Source: CAD feature listing. Evaluate the final solid. Frame: model axes, mm. Give positions to 0.01 mm unless a question says otherwise; leave off trailing zeros. Loops run counter-clockwise (first coordinate to the right, second up) from the corner with the lowest first, then second, coordinate; pieces in that order, holes last. Notation, with made-up numbers: (61, 44.25) -> (69, 44.25) arc R7 ccw to (69, 55.25) -> close; hole circle Ø2 at (-1.75, 14). An arc over 180 degrees is marked (long way). Return JSON: item names as keys, results as strings. Group by question number.
(1) Cut plane D-D on x = 76.2. Return loops of the section in (y, z).
(2) Cut plane C-C on z = -76.2. Return loops of the section in (x, y).
(3) Cut plane B-B on y = 1. Give the number of separate pieces and of enclosed holes in the cut face, then the cut area to 3 significant figures.
(4) Pin query (flat end, axial travel): pin 1 (3 mm diameter, centred on x = 56.5, y = 4.5, fed in from -Z); pin 2 (3 mm diameter, centred on y = 3, z = 1.5, fed in from -X); pin 3 (3 mm diameter, centred on y = 2.5, z = 12, fed in from +X). Return the tip coordinate at first contact, or that it passes through.
(5) Cut plane A-A on x = 0. Return loops of the section in (y, z).
(6) Ray query, line 1 (X direction, y = 3, z = 76.2); line 2 (Z direction, x = 1, y = 3.25); line 3 (Z direction, x = -78, y = 1). Return the intervals inside material, ascending. Write a range as from..to.
```python
from build123d import *

# Parameters (mm, degrees)
BOSS_EXTRUDE1_DEPTH         = 6.35
SKETCH2_R                   = 50.8
CUT_EXTRUDE1_DEPTH          = 6.35
FILLET1_R                   = 50.8
F_1_2_20_TAPPED_HOLE1_D     = 11.50874
F_1_2_20_TAPPED_HOLE1_DEPTH = 29.21
F_1_2_20_TAPPED_HOLE1_TIP   = 3.45757432
CHAMFER1_SIZE               = 2.54


with BuildPart() as part:
    # Sketch1 → Boss-Extrude1 (new body)
    with BuildSketch(Plane(origin=(0, 0, 0), x_dir=(1, 0, 0), z_dir=(0, 1, 0))):
        with BuildLine():
            Line((-45.539487758, 63.5), (45.539487758, 63.5))
            Line((45.539487758, 63.5), (67.219743879, 85.180256121))
            ThreePointArc((67.219743879, 85.180256121), (85.180256121, 85.180256121), (85.180256121, 67.219743879))
            Line((85.180256121, 67.219743879), (63.5, 45.539487758))
            Line((63.5, 45.539487758), (63.5, -45.539487758))
            Line((63.5, -45.539487758), (85.180256121, -67.219743879))
            ThreePointArc((85.180256121, -67.219743879), (85.180256121, -85.180256121), (67.219743879, -85.180256121))
            Line((67.219743879, -85.180256121), (45.539487758, -63.5))
            Line((45.539487758, -63.5), (-45.539487758, -63.5))
            Line((-45.539487758, -63.5), (-67.219743879, -85.180256121))
            ThreePointArc((-67.219743879, -85.180256121), (-85.180256121, -85.180256121), (-85.180256121, -67.219743879))
            Line((-85.180256121, -67.219743879), (-63.5, -45.539487758))
            Line((-63.5, -45.539487758), (-63.5, 45.539487758))
            Line((-63.5, 45.539487758), (-85.180256121, 67.219743879))
            ThreePointArc((-85.180256121, 67.219743879), (-85.180256121, 85.180256121), (-67.219743879, 85.180256121))
            Line((-67.219743879, 85.180256121), (-45.539487758, 63.5))
        make_face()
    extrude(amount=BOSS_EXTRUDE1_DEPTH)

    # Sketch2 → Cut-Extrude1 (cut)
    with BuildSketch(Plane(origin=(0, 6.35, 0), x_dir=(1, 0, 0), z_dir=(0, 1, 0))):
        Circle(SKETCH2_R)
    extrude(amount=-CUT_EXTRUDE1_DEPTH, mode=Mode.SUBTRACT)

    # Fillet1
    fillet1_edges = [part.edges().sort_by_distance(p)[0] for p in [
        (-63.5, 3.175, 45.539487758),
        (-63.5, 3.175, -45.539487758),
        (-45.539487758, 3.175, -63.5),
        (45.539487758, 3.175, -63.5),
        (63.5, 3.175, -45.539487758),
        (63.5, 3.175, 45.539487758),
        (45.539487758, 3.175, 63.5),
        (-45.539487758, 3.175, 63.5),
    ]]
    fillet(fillet1_edges, radius=FILLET1_R)

    # 1/2-20 Tapped Hole1
    with Locations(Plane(origin=(-76.2, 6.35, -76.2), x_dir=(0, 0, 1), z_dir=(0, 1, 0))):
        with Locations((0, 0), (0, 152.4), (152.4, 152.4), (152.4, 0)):
            Hole(F_1_2_20_TAPPED_HOLE1_D / 2, depth=F_1_2_20_TAPPED_HOLE1_DEPTH)
            with Locations((0, 0, -(F_1_2_20_TAPPED_HOLE1_DEPTH + F_1_2_20_TAPPED_HOLE1_TIP / 2))):  # 118° drill point
                Cone(0, F_1_2_20_TAPPED_HOLE1_D / 2, F_1_2_20_TAPPED_HOLE1_TIP, mode=Mode.SUBTRACT)

    # Chamfer1
    chamfer1_edges = [part.edges().sort_by_distance(p)[0] for p in [
        (-50.8, 0, 0),
        (-50.8, 6.35, 0),
    ]]
    chamfer(chamfer1_edges, length=CHAMFER1_SIZE)


solid = part.part
```
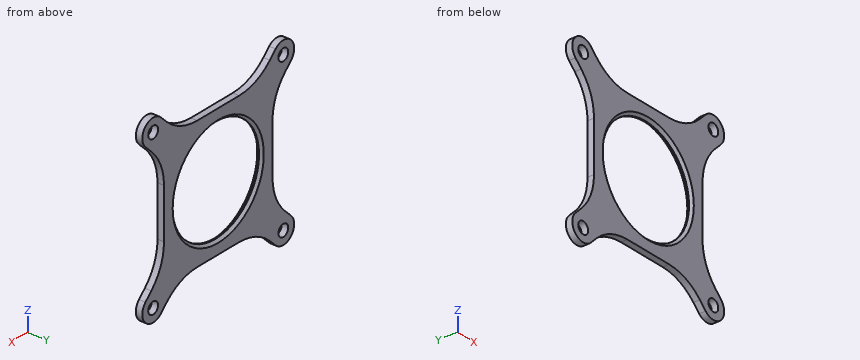
Answers:
{
 "1": {"outline": "(0, -88.9) -> (6.35, -88.9) -> (6.35, -81.95) -> (0, -81.95) -> close; (0, -70.45) -> (6.35, -70.45) -> (6.35, -58.1) -> (0, -58.1) -> close; (0, 58.1) -> (6.35, 58.1) -> (6.35, 70.45) -> (0, 70.45) -> close; (0, 81.95) -> (6.35, 81.95) -> (6.35, 88.9) -> (0, 88.9) -> close"},
 "2": {"outline": "(-88.9, 0) -> (-81.95, 0) -> (-81.95, 6.35) -> (-88.9, 6.35) -> close; (-70.45, 0) -> (-58.1, 0) -> (-58.1, 6.35) -> (-70.45, 6.35) -> close; (58.1, 0) -> (70.45, 0) -> (70.45, 6.35) -> (58.1, 6.35) -> close; (81.95, 0) -> (88.9, 0) -> (88.9, 6.35) -> (81.95, 6.35) -> close"},
 "3": {"separate pieces": "1", "enclosed holes": "5", "area": "11,000 mm²"},
 "4": {"pin 1": "z = -76.11", "pin 2": "x = -63.5", "pin 3": "x = 63.5"},
 "5": {"outline": "(0, -63.5) -> (6.35, -63.5) -> (6.35, -53.34) -> (3.81, -50.8) -> (2.54, -50.8) -> (0, -53.34) -> close; (0, 53.34) -> (2.54, 50.8) -> (3.81, 50.8) -> (6.35, 53.34) -> (6.35, 63.5) -> (0, 63.5) -> close"},
 "6": {"line 1": "-88.9..-81.95, -70.45..-58.1, 58.1..70.45, 81.95..88.9", "line 2": "-63.5..-50.79, 50.79..63.5", "line 3": "-88.77..-81.67, -70.73..-60.04, 60.04..70.73, 81.67..88.77"}
}
